Input: part model. Units: mm. Frame: model coordinates. Round coordinates to 2 decimals unless told otherwise and drop trailing zeros. Loops run counter-clockwise (first coordinate to the right, second up) from the corner with the lowest first, then second, coordinate; pieces in that order, holes last. Notation, with made-up numbers: (-37, 19) -> (-21, 19) arc R10 ccw to (-21, 23) -> close; hole circle Ø7 at (86, 54). An arc over 180 degrees is marked (long way). One line per question, with ' | ' between items. Start each with the question number.
Q1. Material intervals for L1, parallel to Y at x = 2.5, z = 1.3; L2, parallel to Y at x = -50.8, z = 0.6; L3, parallel to X at y = -49.5, z = 0.6, sorted ascending.
Q2. Cut plane C-C on z = 1. Return loops of the section in (x, y) (3 decimals).
Q3. Cut plane A-A on x = -50.8. Return loops of the section in (y, z).
Q4. Contact query for a flat-ended pin moving along its axis: P1, Ø5, axis at x = 50.8, y = 0, coming from the +Z side. Output: stop coordinate, or through.
Q5. Cut plane D-D on y = 35. Return loops of the section in (x, z).
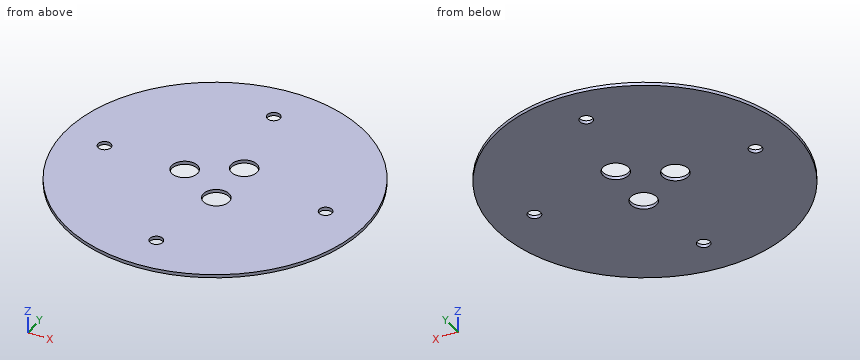
from build123d import *

# Parameters (mm, degrees)
SKETCH1_R           = 69.85
BOSS_EXTRUDE1_DEPTH = 1.524
SKETCH2_R           = 6
CUT_EXTRUDE1_DEPTH  = 2
CUT_EXTRUDE2_REACH  = 100.795
SKETCH3_R           = 3
CIRPATTERN1_COUNT   = 4


with BuildPart() as part:
    # Sketch1 → Boss-Extrude1 (new body)
    with BuildSketch(Plane.XY):
        with Locations(Location((0, 0, 0), (0, 0, 180))):
            Circle(SKETCH1_R)
    extrude(amount=BOSS_EXTRUDE1_DEPTH)

    # Sketch2 → Cut-Extrude1 (cut)
    with BuildSketch(Plane.XY.offset(1.524)):
        with Locations((-13.97, 0)):
            Circle(SKETCH2_R)
        with Locations((6.985, 12.098374891)):
            Circle(SKETCH2_R)
        with Locations((6.985, -12.098374891)):
            Circle(SKETCH2_R)
    extrude(amount=-CUT_EXTRUDE1_DEPTH, mode=Mode.SUBTRACT)

    # Sketch3 → Cut-Extrude2 (cut, up to next)
    with BuildSketch(Plane.XY.offset(1.524), mode=Mode.PRIVATE) as cut_extrude2_sk1:
        with Locations((50.8, 0)):
            Circle(SKETCH3_R)
    cut_extrude2_tool1 = extrude(cut_extrude2_sk1.sketch, amount=-CUT_EXTRUDE2_REACH, mode=Mode.PRIVATE) & part.part
    cut_extrude2 = cut_extrude2_tool1.solids().sort_by_distance((50.8, 0, 1.524))[0]
    add(cut_extrude2, mode=Mode.SUBTRACT)

    # CirPattern1: Cut-Extrude2 ×4 about axis
    cirpattern1_axis = Axis((0, 0, 0), (0, 0, 1))
    for i in range(1, CIRPATTERN1_COUNT):
        add(cut_extrude2.rotate(cirpattern1_axis, i * 360 / CIRPATTERN1_COUNT), mode=Mode.SUBTRACT)


solid = part.part
Results:
1) L1: -69.81 to -52.46, -49.14 to -16.08, -8.11 to 8.11, 16.08 to 49.14, 52.46 to 69.81 | L2: -47.94 to -3, 3 to 47.94 | L3: -49.28 to -2.7, 2.7 to 49.28
2) outline: circle Ø139.7 at (0, 0); hole circle Ø6 at (-50.8, 0); hole circle Ø12 at (-13.97, 0); hole circle Ø6 at (0, -50.8); hole circle Ø6 at (0, 50.8); hole circle Ø12 at (6.985, -12.098); hole circle Ø12 at (6.985, 12.098); hole circle Ø6 at (50.8, 0)
3) outline: (-47.94, 0) -> (-3, 0) -> (-3, 1.52) -> (-47.94, 1.52) -> close; (3, 0) -> (47.94, 0) -> (47.94, 1.52) -> (3, 1.52) -> close
4) P1: through
5) outline: (-60.45, 0) -> (60.45, 0) -> (60.45, 1.52) -> (-60.45, 1.52) -> close
